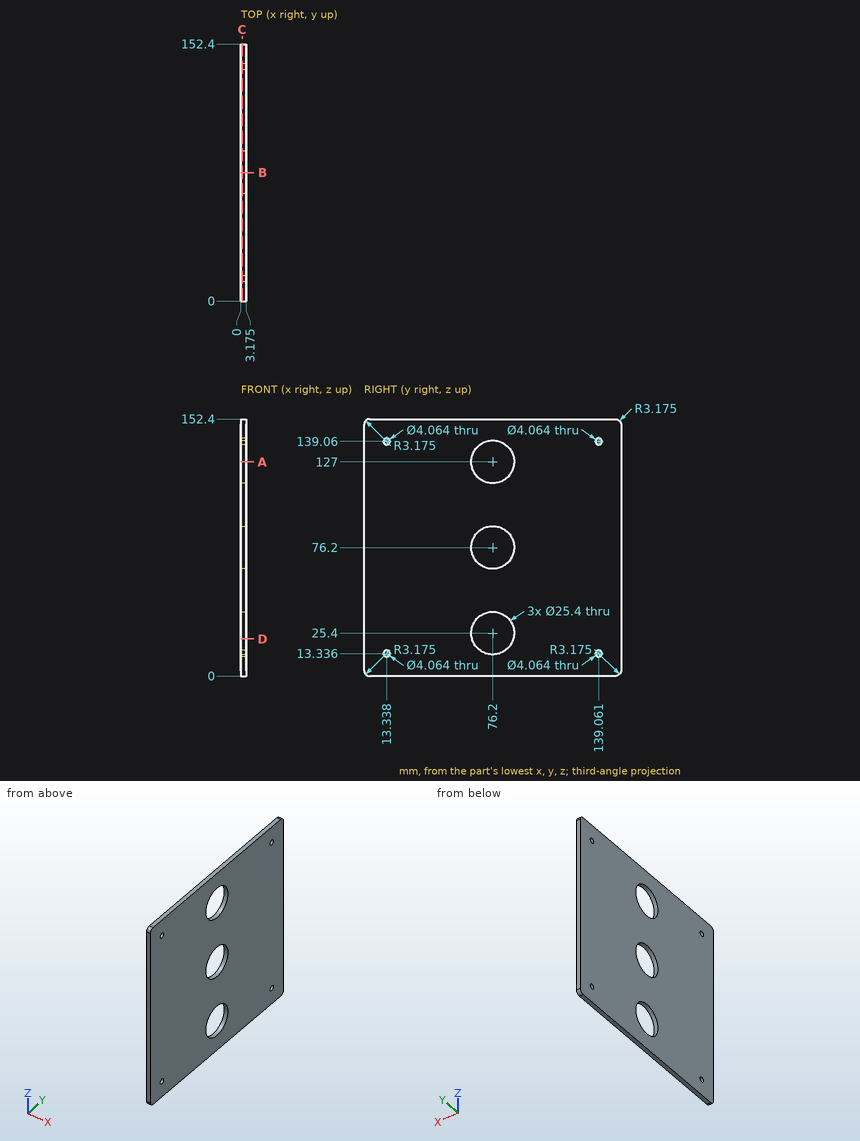
The figure shows three views and two pictorial views of one solid part (mm, origin at its lowest corner). Answer the questions. Give positions to 0.01 mm unless a question says otherwise; leave off trailing zeros. Write each loop counter-clockwise with the first axis right and the second up, starting at its lowest first coordinate (ties: lowest second). Pieces come first, ordered by that corner, then holes. Notation, with made-up numbers: (52.25, 19.5) - (110.25, 19.5) arc R25 ccw to (110.25, 46.5) - close; hole circle Ø11 at (12, 19.5). An arc over 180 degrees is marked (long way). Return JSON: item names as keys, results as strings.
Q1. A cutting plane is placed at D-D, the plane z = 22. Determine the outline of the cut face in (x, y) (1 decimal).
Reply:
{"outline": "(0, 0) - (3.2, 0) - (3.2, 64) - (0, 64) - close; (0, 88.4) - (3.2, 88.4) - (3.2, 152.4) - (0, 152.4) - close"}
Q2. Consider line 1 along Y through (x, z) = (1.9, 76.2); line 2 along Z through (x, y) = (1, 87.5) (1 decimal); line 3 along Y through (x, z) = (2.3, 125.5). Determine where each line is inside the solid, lowest interval first. Write a range as [from, to].
Reply:
{"line 1": "[0, 63.5], [88.9, 152.4]", "line 2": "[0, 19.6], [31.2, 70.4], [82, 121.2], [132.8, 152.4]", "line 3": "[0, 63.59], [88.81, 152.4]"}
Q3. A cutting plane is placed at A-A, the plane z = 127. Determine the outline of the cut face in (x, y) (1 decimal).
Reply:
{"outline": "(0, 0) - (3.2, 0) - (3.2, 63.5) - (0, 63.5) - close; (0, 88.9) - (3.2, 88.9) - (3.2, 152.4) - (0, 152.4) - close"}
Q4. A cutting plane is placed at B-B, the plane y = 76.2. Determine the outline of the cut face in (x, z) (1 decimal).
Reply:
{"outline": "(0, 0) - (3.2, 0) - (3.2, 12.7) - (0, 12.7) - close; (0, 38.1) - (3.2, 38.1) - (3.2, 63.5) - (0, 63.5) - close; (0, 88.9) - (3.2, 88.9) - (3.2, 114.3) - (0, 114.3) - close; (0, 139.7) - (3.2, 139.7) - (3.2, 152.4) - (0, 152.4) - close"}
Q5. A cutting plane is placed at C-C, the plane x = 0.8. Count the separate pieces of the cut face and the enclosed holes in it, and give its area (3 significant figures).
Reply:
{"separate pieces": "1", "enclosed holes": "7", "area": "21,600 mm²"}
